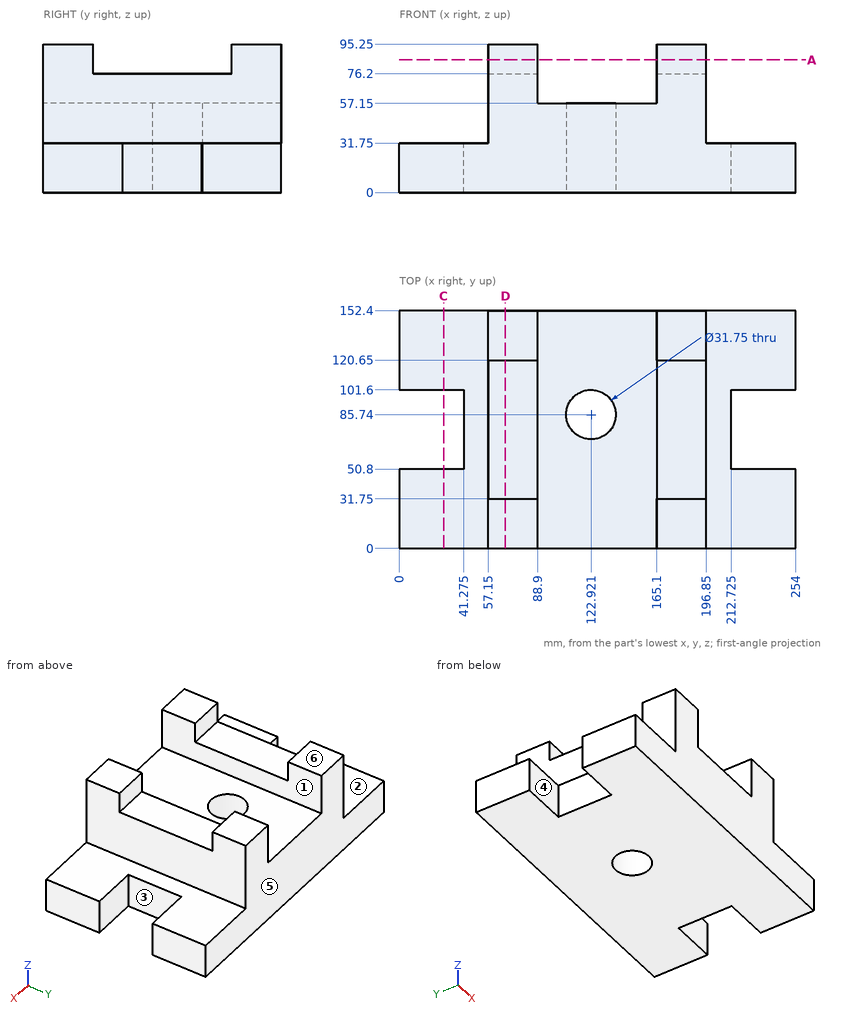
Drawing for the job (mm, zero at the part's lowest x, y, z). A direction names the side the tool comes from. Give positions to 0.01 mm unless a question says otherwise; leave off trailing zeros. Loops run counter-clockwise (first coordinate to the right, second up) from the corner with the lowest first, then second, coordinate; pieces in that order, holes last. Notation, with made-up numbers: M 41,-7 L 61,-7 A31 cw 61,32 Z; hole C -23.5,-29 d7. An arc over 180 degrees is marked long. Use one line per item in the form item = value.
Item 1: Slice it at A-A (z = 85). List the corners of the cut face in (x, y).
Determined:
outline = M 57.15,0 L 88.9,0 L 88.9,31.75 L 57.15,31.75 Z; M 57.15,120.65 L 88.9,120.65 L 88.9,152.4 L 57.15,152.4 Z; M 165.1,0 L 196.85,0 L 196.85,31.75 L 165.1,31.75 Z; M 165.1,120.65 L 196.85,120.65 L 196.85,152.4 L 165.1,152.4 Z
Item 2: Which spindle directions (+Z, -Z, +X, -X, +Y, -Y) get a long thin tool onto all of the face, cutting with end or side? Do the marked faces 1, 2 and 3. Say none if no direction does.
Determined:
face_1 = +Z, +Y, -Y
face_2 = +Z, -X, +Y, -Y
face_3 = +Z, -Z, +X
Item 3: Drill centre lines: probe 1 along X at (y, z) = (129.5, 73.5); probe 2 along Y at (x, z) = (65, 88); probe 3 along Z at (x, y) = (90, 65). Where is each one in solid material? Low to high. Write a range as from..to.
Determined:
probe_1 = 57.15..88.9, 165.1..196.85
probe_2 = 0..31.75, 120.65..152.4
probe_3 = 0..57.15
Item 4: Slice it at C-C (x = 28.5). List the corners of the cut face in (y, z), plus the area to 3 significant figures.
Determined:
outline = M 0,0 L 50.8,0 L 50.8,31.75 L 0,31.75 Z; M 101.6,0 L 152.4,0 L 152.4,31.75 L 101.6,31.75 Z
area = 3,230 mm2
Item 5: Two-plate mould, pull along Y, no slides. Class the marked faces 4, 5 and 6: pulls with the +Y half, pulls with the -Y half, needs draft (parallel to the pull), parting line crosses it, or undercut.
Determined:
face_4 = undercut
face_5 = pulls with the +Y half
face_6 = needs draft
Item 6: Flat gauge pins, fed straight in: pin 1 (19 mm diameter, centred on y = 99, z = 55.5, fed in from +X); pin 2 (2 mm diameter, centred on y = 29.5, z = 37, fed in from -X); pin 3 (9.5 mm diameter, centred on x = 72.5, y = 95, fed in from +Z); pin 4 (4 mm diameter, centred on x = 179.5, z = 13, fed in from -Y). Where does each tip first touch, or does it go through?
Determined:
pin_1 = 196.85
pin_2 = 57.15
pin_3 = 76.2
pin_4 = 0
Item 7: Slice it at D-D (x = 68). List the corners of the cut face in (y, z), plus the area to 3 significant figures.
Determined:
outline = M 0,0 L 152.4,0 L 152.4,95.25 L 120.65,95.25 L 120.65,76.2 L 31.75,76.2 L 31.75,95.25 L 0,95.25 Z
area = 12,800 mm2
